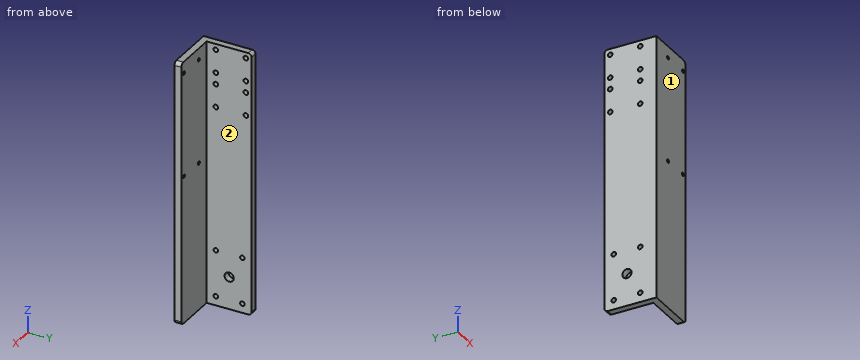
```python
from build123d import *

# Parameters (mm, degrees)
BOSS_EXTRUDE1_DEPTH = 228
FILLET1_R           = 3
SKETCH5_R           = 2
CUT_EXTRUDE2_DEPTH  = 46
SKETCH6_R           = 2
CUT_EXTRUDE3_DEPTH  = 46
SKETCH7_R           = 4
CUT_EXTRUDE4_DEPTH  = 46
SKETCH8_R           = 1.5
CUT_EXTRUDE5_DEPTH  = 7


with BuildPart() as part:
    # Sketch2 → Boss-Extrude1 (new body)
    with BuildSketch(Plane.XY):
        Polygon((82.969208633, 26.8), (82.969208633, -12.2), (121.969208633, -12.2), (121.969208633, -18.2), (82.969208633, -18.2), (76.969208633, -18.2), (76.969208633, -12.2), (76.969208633, 26.8), align=None)
    extrude(amount=BOSS_EXTRUDE1_DEPTH)

    # Fillet1
    fillet1_edges = [part.edges().sort_by_distance(p)[0] for p in [
        (79.969208633, 26.8, 0),
        (121.969208633, -15.2, 228),
        (79.969208633, 26.8, 228),
        (121.969208633, -15.2, 0),
    ]]
    fillet(fillet1_edges, radius=FILLET1_R)

    # Sketch5 → Cut-Extrude2 (cut, through all)
    with BuildSketch(Plane.ZY.offset(-76.969208633)):
        with Locations((223, 21.8)):
            Circle(SKETCH5_R)
        with Locations((223, -4.2)):
            Circle(SKETCH5_R)
        with Locations((203, 21.8)):
            Circle(SKETCH5_R)
        with Locations((203, -4.2)):
            Circle(SKETCH5_R)
    cut_extrude2 = extrude(amount=-CUT_EXTRUDE2_DEPTH, mode=Mode.SUBTRACT)

    # Mirror1: Cut-Extrude2 across plane
    add(cut_extrude2.mirror(Plane.XY.offset(198)), mode=Mode.SUBTRACT)

    # Sketch6 → Cut-Extrude3 (cut, through all)
    with BuildSketch(Plane.ZY.offset(-76.969208633)):
        with Locations((8, 18.8)):
            Circle(SKETCH6_R)
        with Locations((48, 18.8)):
            Circle(SKETCH6_R)
        with Locations((8, -4.2)):
            Circle(SKETCH6_R)
        with Locations((48, -4.2)):
            Circle(SKETCH6_R)
    extrude(amount=-CUT_EXTRUDE3_DEPTH, mode=Mode.SUBTRACT)

    # Sketch7 → Cut-Extrude4 (cut, through all)
    with BuildSketch(Plane.ZY.offset(-76.969208633)):
        with Locations((28, 7.3)):
            Circle(SKETCH7_R)
    extrude(amount=-CUT_EXTRUDE4_DEPTH, mode=Mode.SUBTRACT)

    # Sketch8 → Cut-Extrude5 (cut, through all)
    with BuildSketch(Plane(origin=(0, -12.2, 0), x_dir=(1, 0, 0), z_dir=(0, 1, 0))):
        with Locations((94.969208633, -218)):
            Circle(SKETCH8_R)
        with Locations((117.969208633, -218)):
            Circle(SKETCH8_R)
        with Locations((117.969208633, -128)):
            Circle(SKETCH8_R)
        with Locations((94.969208633, -128)):
            Circle(SKETCH8_R)
    extrude(amount=-CUT_EXTRUDE5_DEPTH, mode=Mode.SUBTRACT)


solid = part.part
```
The listing builds one solid part. Answer for the finished solid, in the listing's coordinates (mm). Face numbers are marked on the shaded views. A direction names the side the tool comes from. Coordinates: 2 decimals unless noted, no trailing zeros. Write each loop counter-clockwise with the first axis right and the second up, starting at its lowest first coordinate (ties: lowest second). Pieces come first, ordered by that corner, then holes. Notation, with made-up numbers: (-35.75, -1) -> (-30.75, -1) arc R22 cw to (-30.75, 19) -> close; hole circle Ø2 at (86, 17.25). An arc over 180 degrees is marked (long way). Write each question's results on one line, items separated by ' | '. Start each with the question number.
1) A cutting plane is placed at D-D (x = 91). Determine the outline of the cut face in (y, z).
2) A tool of negligible diameter and unlimited length cuts with its end or side. For the marked faces 1 and 2, from which of +Z, -Z, +X, -X, +Y, -Y can it reach the whole face along a straight path? Write none if from no direction.
3) A cutting plane is placed at C-C (z = 173). Determine the outline of the cut face in (x, y).
4) Straight lines are drawn through the part: probe 1 along Y at (x, z) = (80.9, 48); probe 2 along Y at (x, z) = (80.2, 173); probe 3 along X at (y, z) = (-14.3, 128). For each, find the intervals that lie inside material, in ascending order.
5) A cutting plane is placed at A-A (z = 28). Determine the outline of the cut face in (x, y), then the cut area to 3 significant figures.
6) Flat-ended cylindrical pins translate along their axes: pin 1 Ø2.5 at (y, z) = (21.8, 203) entering from +X; pin 2 Ø3 at (y, z) = (15, 134.5) entering from +X; pin 3 Ø8 at (x, z) = (88, 98.5) entering from +Y. Find the tip coordinate at first contact, or state that the pin passes through.
7) A cutting plane is placed at B-B (y = 7.3). Determine the outline of the cut face in (x, z), then the cut area to 3 significant figures.
Values follow:
1) outline: (-18.2, 0) -> (-12.2, 0) -> (-12.2, 228) -> (-18.2, 228) -> close
2) face 1: +Z, -Z, +X, -X, -Y | face 2: +Z, -Z, +X, +Y
3) outline: (76.97, -18.2) -> (121.97, -18.2) -> (121.97, -12.2) -> (82.97, -12.2) -> (82.97, -6.2) -> (76.97, -6.2) -> close; (76.97, -2.2) -> (82.97, -2.2) -> (82.97, 19.8) -> (76.97, 19.8) -> close; (76.97, 23.8) -> (82.97, 23.8) -> (82.97, 26.8) -> (76.97, 26.8) -> close
4) probe 1: -18.2 to -6.2, -2.2 to 16.8, 20.8 to 26.8 | probe 2: -18.2 to -6.2, -2.2 to 19.8, 23.8 to 26.8 | probe 3: 76.97 to 93.47, 96.47 to 116.47, 119.47 to 121.97
5) outline: (76.97, -18.2) -> (121.97, -18.2) -> (121.97, -12.2) -> (82.97, -12.2) -> (82.97, 3.3) -> (76.97, 3.3) -> close; (76.97, 11.3) -> (82.97, 11.3) -> (82.97, 26.8) -> (76.97, 26.8) -> close | area: 456 mm²
6) pin 1: through | pin 2: x = 82.97 | pin 3: y = -12.2
7) outline: (76.97, 0) -> (82.97, 0) -> (82.97, 24) -> (76.97, 24) -> close; (76.97, 32) -> (82.97, 32) -> (82.97, 228) -> (76.97, 228) -> close | area: 1,320 mm²
